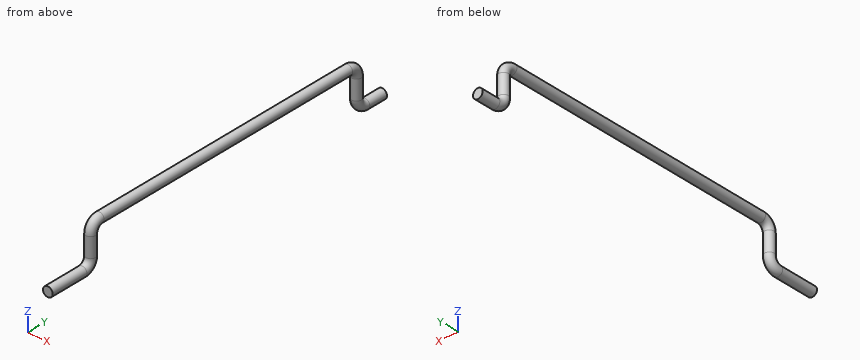
```python
from build123d import *

# Parameters (mm, degrees)
SKETCH2_R = 0.5


with BuildPart() as part:
    # Sweep1: sweep along a path in Sketch1
    with BuildLine(Plane(origin=(0, 0, 0), x_dir=(0, 0, -1), z_dir=(1, 0, 0))) as sweep1_path:
        Line((13.22, -2), (13.22, 2))
        ThreePointArc((13.22, 2), (12.927106781, 2.707106781), (12.22, 3))
        Line((12.22, 3), (10.22, 3))
        ThreePointArc((10.22, 3), (9.512893219, 3.292893219), (9.22, 4))
        Line((9.22, 4), (9.22, 33))
        ThreePointArc((9.22, 33), (9.512893219, 33.707106781), (10.22, 34))
        Line((10.22, 34), (12.22, 34))
        ThreePointArc((12.22, 34), (12.927106781, 34.292893219), (13.22, 35))
        Line((13.22, 35), (13.22, 37))
    # Sketch2 → Sweep1 (sweep)
    with BuildSketch(Plane(origin=(0, -2, 0), x_dir=(1, 0, 0), z_dir=(0, 1, 0))):
        with Locations((0, 13.22)):
            Circle(SKETCH2_R)
    sweep(path=sweep1_path.line)


solid = part.part
```
Geometry: final body of the model. Coordinates: model frame, mm. Round coordinates to 2 decimals unless told otherwise and drop trailing zeros. Order: outer loops, then holes, each group sorted by start corner. A loop starts at its lowest first (then second) coordinate and runs counter-clockwise, first axis right, second up. Notation, with made-up numbers: M 50,47 L 84,47 A24 ccw 84,71 Z; hole C -30,59.25 d3. An arc over 180 degrees is marked long. One line per item, written item: value.
(1) Cut plane C-C (y = 30). Return the cut outline in (x, z), and give its area (3 significant figures).
Result sheet:
outline: C 0,-9.22 d1
area: 0.785 mm2
(2) Cut plane A-A (x = 0). Return the cut outline in (y, z).
Result sheet:
outline: M -2,-13.72 L 2,-13.72 A1.5 ccw 3.5,-12.22 L 3.5,-10.22 A0.5 cw 4,-9.72 L 33,-9.72 A0.5 cw 33.5,-10.22 L 33.5,-12.22 A1.5 ccw 35,-13.72 L 37,-13.72 L 37,-12.72 L 35,-12.72 A0.5 cw 34.5,-12.22 L 34.5,-10.22 A1.5 ccw 33,-8.72 L 4,-8.72 A1.5 ccw 2.5,-10.22 L 2.5,-12.22 A0.5 cw 2,-12.72 L -2,-12.72 Z
(3) Pin query (flat end, axial travel): P1, Ø1.5, axis at y = 19, z = -11.5, coming from the -X side. Return the tip coordinate at first contact, or that it passes through.
Result sheet:
P1: through
(4) Line query: probe 1 along Y at (x, z) = (0.05, -9.85); probe 2 along Y at (x, z) = (0.3, -12.15); probe 3 along Z at (x, y) = (0.1, 28). Output: solid intervals per line, ascending. Write a range as [from, to].
Result sheet:
probe 1: [2.55, 3.66], [33.34, 34.45]
probe 2: [2.6, 3.4], [33.6, 34.4]
probe 3: [-9.71, -8.73]
(5) Cut plane B-B (z = -11.25). Return the cut outline in (x, y).
Result sheet:
outline: C 0,3 d1; C 0,34 d1
